Geometry: final body of the model. Coordinates: model frame, mm. A direction names the side the tool comes from. Round coordinates to 2 decimals unless told otherwise and drop trailing zeros. Loops run counter-clockwise (first coordinate to the right, second up) from the corner with the lowest first, then second, coordinate; pieces in that order, holes last. Notation, with made-up numbers: M 42.5,-28.5 L 54.5,-28.5 A12 cw 54.5,-24.5 Z; hole C -14,66 d1. An arc over 180 degrees is marked long. Return JSON: item names as keys, results as strings.
from build123d import *

# Parameters (mm, degrees)
F0_W      = 71.12
F0_H      = 71.12
F1_DEPTH  = 61.976
F2_W      = 71.12
F2_H      = 51.816
F3_DEPTH  = 10.16
F4_W      = 71.12
F4_H      = 51.816
F5_DEPTH  = 10.16
F7_DEPTH  = 76.2
F9_DEPTH  = 76.2
F10_R     = 19.05
F11_DEPTH = 76.2


with BuildPart() as f1:
    # F0 (on Top) → F1 (new body)
    with BuildSketch(Plane.XY):
        with Locations((-18.7232699245, 27.0034961376)):
            Rectangle(F0_W, F0_H)
    extrude(amount=F1_DEPTH)

    # F2 (on face) → F3 (cut)
    with BuildSketch(Plane.XZ.offset(8.5565038624)):
        with Locations((-18.7232699245, 36.068)):
            Rectangle(F2_W, F2_H)
    extrude(amount=-F3_DEPTH, mode=Mode.SUBTRACT)

    # F4 (on face) → F5 (cut)
    with BuildSketch(Plane(origin=(0, 62.5634961376, 0), x_dir=(-1, 0, 0), z_dir=(0, 1, 0))):
        with Locations((18.7232699245, 36.068)):
            Rectangle(F4_W, F4_H)
    extrude(amount=-F5_DEPTH, mode=Mode.SUBTRACT)

    # F6 (on face) → F7 (cut)
    with BuildSketch(Plane.XZ.offset(-1.6034961376)):
        Polygon((-33.9632699245, 61.976), (-54.2832699245, 61.976), (-54.2832699245, 41.656), align=None)
    extrude(amount=-F7_DEPTH, mode=Mode.SUBTRACT)

    # F8 (on face) → F9 (cut)
    with BuildSketch(Plane.XZ.offset(-1.6034961376)):
        Polygon((-21.3656260499, 61.976), (16.7347530496, 23.8756209005), (16.8367300755, 10.16), (16.8367300755, 61.976), align=None)
    extrude(amount=-F9_DEPTH, mode=Mode.SUBTRACT)

    # F10 (on face) → F11 (cut)
    with BuildSketch(Plane(origin=(20.3051869751, 0, 20.3051869751), x_dir=(0.7071067812, 0, -0.7071067812), z_dir=(0.7071067812, 0, 0.7071067812))):
        with Locations((-33.9787192643, 26.5149436891)):
            Circle(F10_R)
    extrude(amount=-F11_DEPTH, mode=Mode.SUBTRACT)


solid = f1.part
Q1. Pin query (flat end, axial travel): pin 1 (12 mm diameter, centred on x = -4, z = 44, fed in from +Y); pin 2 (5 mm diameter, centred on x = -30, y = 58, fed in from +Z); pin 3 (3 mm diameter, centred on x = -46, y = 9.5, fed in from +Z). Return the tip coordinate at first contact, or that it passes through.
Determined:
{"pin 1": "stops at y = 52.4", "pin 2": "stops at z = 10.16", "pin 3": "stops at z = 51.44"}
Q2. Material intervals for L1, parallel to X at y = 24, z = 27.5; L2, parallel to Y at x = -3, z = 20.5; L3, parallel to Y at x = -5, z = 29, sorted ascending.
Determined:
{"L1": "x = -54.28 to -47.26, 6.15 to 13.11", "L2": "y = 1.6 to 18.67, 34.36 to 52.4", "L3": "y = 1.6 to 10.26, 42.77 to 52.4"}
Q3. Section query B-B (x = 11). Output: boundary loops of the cut face in (y, z), plus the area to 3 significant figures.
Determined:
{"outline": "M -8.56,0 L 62.56,0 L 62.56,10.16 L 52.4,10.16 L 52.4,29.61 L 1.6,29.61 L 1.6,10.16 L -8.56,10.16 Z", "area": "1,710 mm^2"}
Q4. Section query A-A (y = 43). Output: boundary loops of the cut face in (x, z), plus the area to 3 significant figures.
Determined:
{"outline": "M -54.28,7.27 L -10.47,51.08 L -21.37,61.98 L -33.96,61.98 L -54.28,41.66 Z; M -34.55,0 L 16.84,0 L 16.84,10.16 L 16.73,23.88 L 3.03,37.58 Z", "area": "2,300 mm^2"}
Q5. Pull-direction query (Y, two-part tool) for faces 4 (the flat face through (-19, 1.603, 31)), 5 (the flat face through (-18, 58, 10.16)), 6 (the cylindrical face through (-35.3, 27.35, 39.67)); classes: pulls with the +Y half, pulls with the -Y half, needs draft (parallel to the pull), parting line crosses it, or undercut.
Determined:
{"face 4": "pulls with the -Y half", "face 5": "needs draft", "face 6": "undercut"}
Q6. Reachability of faces 1 (the flat face through (-26, 52.403, 31)), 2 (the flat face through (-28, 27, 61.976)), 3 (the flat face through (-19, -4, 10.16)) from +Z, -Z, +X, -X, +Y, -Y: full face, straight path, thin tool, end or side. Return the list, or none.
Determined:
{"face 1": "+Z, +X, -X, +Y", "face 2": "+Z, +X, -X, +Y, -Y", "face 3": "+Z, +X, -X, -Y"}
Q7. Section query C-C (y = 53.5). Output: boundary loops of the cut face in (x, z), plus the area to 3 significant figures.
Determined:
{"outline": "M -54.28,0 L 16.84,0 L 16.84,10.16 L -54.28,10.16 Z", "area": "723 mm^2"}
